Check sheet for the modelled part. Datum: model origin and axes. Units: mm. A direction names the side the tool comes from. Give positions to 0.01 mm unless a question says otherwise; leave off trailing zeros. Write each loop counter-clockwise with the first axis right and the second up, starting at its lowest first coordinate (ties: lowest second). Pieces come first, ordered by that corner, then holes. Notation, with made-up numbers: M 20,11 L 25,11 A14 cw 25,31 Z; hole C 16.25,17 d4. An arc over 180 degrees is marked long. Write item = value, one per line. Start each with the question number.
1) Cross-section at D-D, the plane x = -278. Record the cut outline in (y, z), plus the area to 3 significant figures.
2) Access from +Z, -Z, +X, -X, +Y, -Y to the whole of each face (thin tool, end or side, straight path). Record for faces 1 (the flat face through (-23, 3, -15)), 2 (the flat face through (-240, 30, -3)), 3 (the flat face through (237, 29.235, -1)).
3) Scan lines: line 1 along Y through (x, z) = (4, 7.5); line 2 along Z through (x, y) = (37.5, 28.5); line 3 along Y through (x, z) = (205.5, 8). Record each from-to range of solid material in increasing order. Write a range as [from, to].
4) Cross-section at B-B, the plane z = -5.5. Record the cut outline in (x, y).
5) Mould release check, pull along X, two halves, no side actions. Record for faces 4 (the flat face through (-40, -32, 0)), 5 (the flat face through (-40, 35, 0)), 6 (the flat face through (40, -33, 0)): released by +X, released by -X, zero draft, split by the parting line, or undercut.
6) Go/stop test with flat-tipped pins: pin 1 (24 mm diameter, centred on x = -16, z = 3, fed in from +Y); pin 2 (5 mm diameter, centred on x = -13.5, y = -27, fed in from -Z); pin 3 (1.5 mm diameter, centred on x = -80.5, y = -0.5, fed in from +Z); pin 4 (1.5 mm diameter, centred on x = -237.5, y = 31, fed in from +Z). Record where each tip stops, or that it passes through.
7) Cross-section at C-C, the plane y = -31. Record the cut outline in (x, z), plus the area to 3 significant figures.
8) Cross-section at A-A, the plane z = 27. Record the cut outline in (x, y).
```python
from build123d import *

# Parameters (mm, degrees)
BOSS_EXTRUDE1_DEPTH = 15
SKETCH2_W           = 75
SKETCH2_H           = 75
BOSS_EXTRUDE2_DEPTH = 20
SKETCH3_W           = 75
SKETCH3_H           = 75
BOSS_EXTRUDE3_DEPTH = 20


with BuildPart() as part:
    # Sketch1 → Boss-Extrude1 (new body, symmetric)
    with BuildSketch(Plane.XY):
        Polygon((-40, -25), (-40, -40), (40, -40), (40, -25), (200, 33.235237483), (200, 29.235237483), (257, 29.235237483), (257, 49.235237483), (200, 49.235237483), (200, 45.235237483), (40, 30), (40, 40), (-40, 40), (-40, 30), (-240, 29.511312334), (-240, 33.511312334), (-297, 33.511312334), (-297, 13.511312334), (-240, 13.511312334), (-240, 17.511312334), align=None)
    extrude(amount=BOSS_EXTRUDE1_DEPTH, both=True)

    # Sketch2 → Boss-Extrude2 (add)
    with BuildSketch(Plane(origin=(0, 33.511312334, 0), x_dir=(1, 0, 0), z_dir=(0, 1, 0))):
        with Locations((-277.5, 3.224825952)):
            Rectangle(SKETCH2_W, SKETCH2_H)
    extrude(amount=-BOSS_EXTRUDE2_DEPTH)

    # Sketch3 → Boss-Extrude3 (add)
    with BuildSketch(Plane(origin=(0, 49.235237483, 0), x_dir=(1, 0, 0), z_dir=(0, 1, 0))):
        with Locations((237.5, 0)):
            Rectangle(SKETCH3_W, SKETCH3_H)
    extrude(amount=-BOSS_EXTRUDE3_DEPTH)


solid = part.part
```
Reply:
q1.outline = M 13.51,-40.72 L 33.51,-40.72 L 33.51,34.28 L 13.51,34.28 Z
q1.area = 1,500 mm2
q2.face_1 = -Z, +Y, -Y
q2.face_2 = none
q2.face_3 = +Z, -Z, +X, -Y
q3.line_1 = [-40, 40]
q3.line_2 = [-15, 15]
q3.line_3 = [29.24, 49.24]
q4.outline = M -315,13.51 L -240,13.51 L -240,17.51 L -40,-25 L -40,-40 L 40,-40 L 40,-25 L 200,33.24 L 200,29.24 L 275,29.24 L 275,49.24 L 200,49.24 L 200,45.24 L 40,30 L 40,40 L -40,40 L -40,30 L -240,29.51 L -240,33.51 L -315,33.51 Z
q5.face_4 = released by -X
q5.face_5 = undercut
q5.face_6 = released by +X
q6.pin_1 = 40
q6.pin_2 = -15
q6.pin_3 = 15
q6.pin_4 = through
q7.outline = M -40,-15 L 40,-15 L 40,15 L -40,15 Z
q7.area = 2,400 mm2
q8.outline = M -315,13.51 L -240,13.51 L -240,33.51 L -315,33.51 Z; M 200,29.24 L 275,29.24 L 275,49.24 L 200,49.24 Z
